Build history of the part. All positions in model axes, mm. Face numbers are marked on the shaded views. Give positions to 0.01 mm unless a question says otherwise; leave off trailing zeros. Loops run counter-clockwise (first coordinate to the right, second up) from the corner with the lowest first, then second, coordinate; pieces in that order, holes last. Notation, with made-up numbers: M 27,40.25 L 56,40.25 A18 ccw 56,71.25 Z; hole C 20.5,20.25 d4. An arc over 180 degrees is marked long. Answer as a JSON object with one key per item and string values. Group by question number.
1. Slice it at A-A (x = 0). List the corners of the cut face in (y, z).
2. Slice it at C-C (y = 20.5). List the corners of the cut face in (x, z).
3. Mould opens along Z. For the marked faces 1, 2, 3 and 4 say: released by +Z, released by -Z, zero draft, split by the parting line, or undercut.
4. Drill centre lines: line 1 along Y through (x, z) = (7.15, 8); line 2 along Z through (x, y) = (-0.25, 12.5); line 3 along Y through (x, z) = (0, 11). Where is each one in solid material? Low to high. Write a range as [from, to].
5. Drop a flat-ended pin along its axis: pin 1 Ø3 at (x, z) = (2.5, 7) entering from -Y. Give the stop position or say it passes through.
6. Slice it at D-D (x = -4). List the corners of the cut face in (y, z), then the cut area to 3 significant figures.
7. Slice it at B-B (y = 9). List the corners of the cut face in (x, z), then the cut area to 3 significant figures.
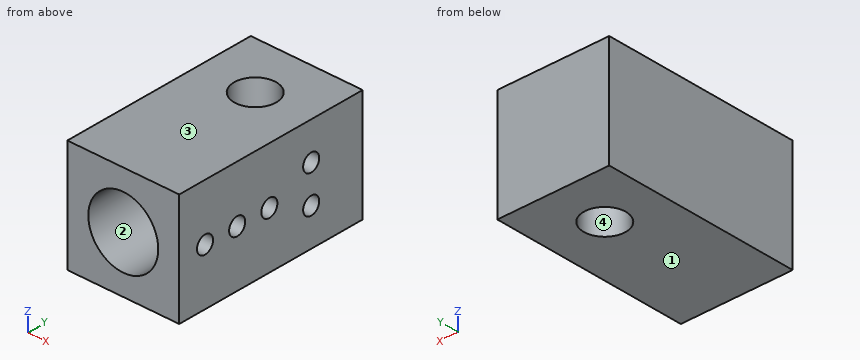
from build123d import *

# Parameters (mm, degrees)
SKETCH1_W           = 16
SKETCH1_H           = 28.5
BOSS_EXTRUDE1_DEPTH = 16
SKETCH2_R           = 5
CUT_EXTRUDE1_DEPTH  = 16
SKETCH3_R           = 3
CUT_EXTRUDE2_DEPTH  = 34.648922717
SKETCH4_R           = 1.25
CUT_EXTRUDE3_DEPTH  = 10
SKETCH6_R           = 1.25
CUT_EXTRUDE4_DEPTH  = 8


with BuildPart() as part:
    # Sketch1 → Boss-Extrude1 (new body)
    with BuildSketch(Plane.XY):
        with Locations((0, 14.25)):
            Rectangle(SKETCH1_W, SKETCH1_H)
    extrude(amount=BOSS_EXTRUDE1_DEPTH)

    # Sketch2 → Cut-Extrude1 (cut)
    with BuildSketch(Plane(origin=(0, 0, 0), x_dir=(-1, 0, 0), z_dir=(0, -1, 0))):
        with Locations(Location((0, -8, 0), (0, 0, 90))):
            Circle(SKETCH2_R)
    extrude(amount=-CUT_EXTRUDE1_DEPTH, mode=Mode.SUBTRACT)

    # Sketch3 → Cut-Extrude2 (cut, through all)
    with BuildSketch(Plane(origin=(0, 0, 0), x_dir=(-1, 0, 0), z_dir=(0, 0, -1))):
        with Locations((0, 20.5)):
            Circle(SKETCH3_R)
    extrude(amount=-CUT_EXTRUDE2_DEPTH, mode=Mode.SUBTRACT)

    # Sketch4 → Cut-Extrude3 (cut)
    with BuildSketch(Plane(origin=(8, 0, 0), x_dir=(0, 0, -1), z_dir=(1, 0, 0))):
        with Locations(Location((-10.666666667, 20.5, 0), (0, 0, 90))):
            Circle(SKETCH4_R)
        with Locations(Location((-5.333333333, 20.5, 0), (0, 0, 90))):
            Circle(SKETCH4_R)
    extrude(amount=-CUT_EXTRUDE3_DEPTH, mode=Mode.SUBTRACT)

    # Sketch6 → Cut-Extrude4 (cut)
    with BuildSketch(Plane(origin=(8, 0, 0), x_dir=(0, 0, -1), z_dir=(1, 0, 0))):
        with Locations(Location((-8, 14, 0), (0, 0, 90))):
            Circle(SKETCH6_R)
        with Locations(Location((-8, 9, 0), (0, 0, 90))):
            Circle(SKETCH6_R)
        with Locations(Location((-8, 4, 0), (0, 0, 90))):
            Circle(SKETCH6_R)
    extrude(amount=-CUT_EXTRUDE4_DEPTH, mode=Mode.SUBTRACT)


solid = part.part
Established:
{
 "1": {"outline": "M 0,0 L 17.5,0 L 17.5,16 L 0,16 L 0,13 L 16,13 L 16,3 L 0,3 Z; M 23.5,0 L 28.5,0 L 28.5,16 L 23.5,16 Z"},
 "2": {"outline": "M -8,0 L -3,0 L -3,16 L -8,16 Z; M 3,0 L 8,0 L 8,4.08 L 3,4.08 Z; M 3,6.58 L 8,6.58 L 8,9.42 L 3,9.42 Z; M 3,11.92 L 8,11.92 L 8,16 L 3,16 Z"},
 "3": {"face 1": "released by -Z", "face 2": "undercut", "face 3": "released by +Z", "face 4": "zero draft"},
 "4": {"line 1": "y = [0, 2.75], [5.25, 7.75], [10.25, 12.75], [15.25, 28.5]", "line 2": "z = [0, 3.01], [12.99, 16]", "line 3": "y = [16, 17.5], [23.5, 28.5]"},
 "5": {"pin 1": "stops at y = 16"},
 "6": {"outline": "M 0,0 L 28.5,0 L 28.5,16 L 0,16 L 0,11 L 16,11 L 16,5 L 0,5 Z", "area": "360 mm^2"},
 "7": {"outline": "M -8,0 L 8,0 L 8,6.75 L 4.84,6.75 A5 cw long 4.84,9.25 L 8,9.25 L 8,16 L -8,16 Z", "area": "170 mm^2"}
}
